```python
from build123d import *

# Parameters (mm, degrees)
EXTRUDE_1_DEPTH                  = 5
HOLE_WIZARD_M2_1_D               = 1.6
HOLE_WIZARD_M2_1_DEPTH           = 6.719311505
HOLE_WIZARD_M2_1_TIP             = 0.480688495
HOLE_WIZARD_M2_2_D               = 1.6
HOLE_WIZARD_M2_2_DEPTH           = 6.719311505
HOLE_WIZARD_M2_2_TIP             = 0.480688495
HOLE_WIZARD_M2_2_ON_FACE_2_D     = 1.6
HOLE_WIZARD_M2_2_ON_FACE_2_DEPTH = 6.719311505
HOLE_WIZARD_M2_2_ON_FACE_2_TIP   = 0.480688495
HOLE_WIZARD_M2_2_ON_FACE_3_D     = 1.6
HOLE_WIZARD_M2_2_ON_FACE_3_DEPTH = 6.719311505
HOLE_WIZARD_M2_2_ON_FACE_3_TIP   = 0.480688495
HOLE_WIZARD_M2_2_ON_FACE_4_D     = 1.6
HOLE_WIZARD_M2_2_ON_FACE_4_DEPTH = 6.719311505
HOLE_WIZARD_M2_2_ON_FACE_4_TIP   = 0.480688495


with BuildPart() as part:
    # 草图1 → 凸台-拉伸1 (new body)
    with BuildSketch(Plane(origin=(0, 0, 0), x_dir=(1, 0, 0), z_dir=(0, 1, 0))):
        Polygon((-112.583302492, 65), (-112.583302492, -65), (0, -130), (112.583302492, -65), (112.583302492, 65), (0, 130), align=None)
        with BuildLine():
            Line((0, -130), (-112.583302492, -65))
            Line((-112.583302492, -65), (-115.333302492, -69.763139721))
            ThreePointArc((-115.333302492, -69.763139721), (-115.832804605, -73.557234946), (-113.503175473, -76.59326674))
            Line((-113.503175473, -76.59326674), (-9.580127019, -136.59326674))
            ThreePointArc((-9.580127019, -136.59326674), (-5.786031793, -137.092768852), (-2.75, -134.763139721))
            Line((-2.75, -134.763139721), (0, -130))
        make_face()
        with BuildLine():
            Line((-115.333302492, 69.763139721), (-112.583302492, 65))
            Line((-112.583302492, 65), (0, 130))
            Line((0, 130), (-2.75, 134.763139721))
            ThreePointArc((-2.75, 134.763139721), (-5.786031793, 137.092768852), (-9.580127019, 136.59326674))
            Line((-9.580127019, 136.59326674), (-113.503175473, 76.59326674))
            ThreePointArc((-113.503175473, 76.59326674), (-115.832804605, 73.557234946), (-115.333302492, 69.763139721))
        make_face()
        with BuildLine():
            Line((112.583302492, 65), (112.583302492, -65))
            Line((112.583302492, -65), (118.083302492, -65))
            ThreePointArc((118.083302492, -65), (121.618836398, -63.535533906), (123.083302492, -60))
            Line((123.083302492, -60), (123.083302492, 60))
            ThreePointArc((123.083302492, 60), (121.618836398, 63.535533906), (118.083302492, 65))
            Line((118.083302492, 65), (112.583302492, 65))
        make_face()
    extrude(amount=EXTRUDE_1_DEPTH)

    # M2 螺纹孔1
    with Locations(Plane(origin=(123.083302492, 0, 0), x_dir=(0, 0, -1), z_dir=(1, 0, 0))):
        with Locations((15, 2.5), (-15, 2.5)):
            Hole(HOLE_WIZARD_M2_1_D / 2, depth=HOLE_WIZARD_M2_1_DEPTH)
            with Locations((0, 0, -(HOLE_WIZARD_M2_1_DEPTH + HOLE_WIZARD_M2_1_TIP / 2))):  # 118° drill point
                Cone(0, HOLE_WIZARD_M2_1_D / 2, HOLE_WIZARD_M2_1_TIP, mode=Mode.SUBTRACT)

    # M2 螺纹孔2
    with Locations(Plane(origin=(-48.551270189, 2.5, 114.09326674), x_dir=(0.866025403784, 0, 0.5), z_dir=(-0.5, 0, 0.866025403784))):
        with Locations((0, 0)):
            Hole(HOLE_WIZARD_M2_2_D / 2, depth=HOLE_WIZARD_M2_2_DEPTH)
            with Locations((0, 0, -(HOLE_WIZARD_M2_2_DEPTH + HOLE_WIZARD_M2_2_TIP / 2))):  # 118° drill point
                Cone(0, HOLE_WIZARD_M2_2_D / 2, HOLE_WIZARD_M2_2_TIP, mode=Mode.SUBTRACT)

    # M2 螺纹孔2 on face 2
    with Locations(Plane(origin=(-74.532032303, 2.5, 99.09326674), x_dir=(0.866025302838, 0, 0.500000174844), z_dir=(-0.500000174844, 0, 0.866025302838))):
        with Locations((0, 0)):
            Hole(HOLE_WIZARD_M2_2_ON_FACE_2_D / 2, depth=HOLE_WIZARD_M2_2_ON_FACE_2_DEPTH)
            with Locations((0, 0, -(HOLE_WIZARD_M2_2_ON_FACE_2_DEPTH + HOLE_WIZARD_M2_2_ON_FACE_2_TIP / 2))):  # 118° drill point
                Cone(0, HOLE_WIZARD_M2_2_ON_FACE_2_D / 2, HOLE_WIZARD_M2_2_ON_FACE_2_TIP, mode=Mode.SUBTRACT)

    # M2 螺纹孔2 on face 3
    with Locations(Plane(origin=(-74.532032303, 2.5, -99.09326674), x_dir=(-0.866025302838, 0, 0.500000174844), z_dir=(-0.500000174844, 0, -0.866025302838))):
        with Locations((0, 0)):
            Hole(HOLE_WIZARD_M2_2_ON_FACE_3_D / 2, depth=HOLE_WIZARD_M2_2_ON_FACE_3_DEPTH)
            with Locations((0, 0, -(HOLE_WIZARD_M2_2_ON_FACE_3_DEPTH + HOLE_WIZARD_M2_2_ON_FACE_3_TIP / 2))):  # 118° drill point
                Cone(0, HOLE_WIZARD_M2_2_ON_FACE_3_D / 2, HOLE_WIZARD_M2_2_ON_FACE_3_TIP, mode=Mode.SUBTRACT)

    # M2 螺纹孔2 on face 4
    with Locations(Plane(origin=(-48.551270189, 2.5, -114.09326674), x_dir=(-0.866025302838, 0, 0.500000174844), z_dir=(-0.500000174844, 0, -0.866025302838))):
        with Locations((0, 0)):
            Hole(HOLE_WIZARD_M2_2_ON_FACE_4_D / 2, depth=HOLE_WIZARD_M2_2_ON_FACE_4_DEPTH)
            with Locations((0, 0, -(HOLE_WIZARD_M2_2_ON_FACE_4_DEPTH + HOLE_WIZARD_M2_2_ON_FACE_4_TIP / 2))):  # 118° drill point
                Cone(0, HOLE_WIZARD_M2_2_ON_FACE_4_D / 2, HOLE_WIZARD_M2_2_ON_FACE_4_TIP, mode=Mode.SUBTRACT)


solid = part.part
```
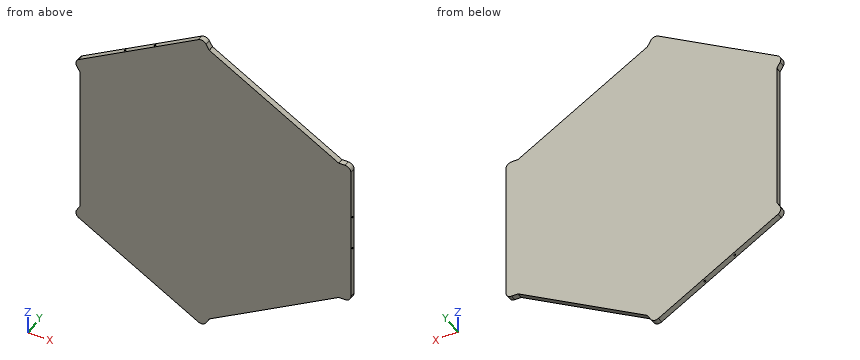
Input: part model. Units: mm. Frame: model coordinates. Round coordinates to 2 decimals unless told otherwise and drop trailing zeros. Write each loop counter-clockwise with the first axis right and the second up, starting at its lowest first coordinate (ties: lowest second). Pieces come first, ordered by that corner, then holes. Notation, with made-up numbers: M -14.75,6.25 L 22.25,6.25 A7 cw 22.25,18.25 Z; hole C -9.5,-9 d10. An arc over 180 degrees is marked long. Write each question's results on one line, items separated by ' | '.
Q1. Section query A-A (y = 4.2). Return loops of the section in (x, z).
Results:
outline: M -115.33,-69.76 A5 ccw -113.5,-76.59 L -9.58,-136.59 A5 ccw -2.75,-134.76 L 0,-130 L 112.58,-65 L 118.08,-65 A5 ccw 123.08,-60 L 123.08,60 A5 ccw 118.08,65 L 112.58,65 L 0,130 L -2.75,134.76 A5 ccw -9.58,136.59 L -113.5,76.59 A5 ccw -115.33,69.76 L -112.58,65 L -112.58,-65 Z
Q2. Pin query (flat end, axial travel): P1, Ø1.5, axis at y = 1.5, z = 43.5, coming from the -X side. Return the tip coordinate at first contact, or that it passes through.
Results:
P1: stops at x = -112.58
Q3. Line query: line 1 along Z through (x, y) = (118.25, 2.5); line 2 along Y through (x, z) = (120.75, 15); line 3 along X through (y, z) = (1.55, 8). Output: solid intervals per line, ascending.
Results:
line 1: z = -65 to -15.8, -14.2 to 14.2, 15.8 to 65 | line 2: y = 0 to 1.7, 3.3 to 5 | line 3: x = -112.58 to 123.08
Q4. Section query B-B (x = -18). Return loops of the section in (y, z).
Results:
outline: M 0,-131.73 L 5,-131.73 L 5,131.73 L 0,131.73 Z
Q5. Section query C-C (x = -100). Return loops of the section in (y, z).
Results:
outline: M 0,-84.39 L 5,-84.39 L 5,84.39 L 0,84.39 Z
